from build123d import *

# Parameters (mm, degrees)
F0_R     = 3.175
F0_R_2   = 20.32
F1_DEPTH = 6.35
F2_R     = 7.62
F3_R     = 26.9875
F3_R_2   = 19.685
F4_DEPTH = 12.7
F5_R     = 0.508


with BuildPart() as f1:
    # F0 (on Top) → F1 (new body)
    with BuildSketch(Plane.XY):
        with BuildLine():
            ThreePointArc((-11.5499308761, 24.3910691239), (-8.0975226707, 25.7440339273), (-4.4922459427, 26.6109917636))
            ThreePointArc((-4.4922459427, 26.6109917636), (-5.8575862517, 27.8922864976), (-6.8692513658, 29.4678511747))
            Line((-6.8692513658, 29.4678511747), (-11.5499308761, 24.3910691239))
        make_face()
        with BuildLine():
            ThreePointArc((4.4922459427, 26.6109917636), (8.0975226707, 25.7440339273), (11.5499308761, 24.3910691239))
            Line((11.5499308761, 24.3910691239), (6.8692513658, 29.4678511747))
            ThreePointArc((6.8692513658, 29.4678511747), (5.8575862517, 27.8922864976), (4.4922459427, 26.6109917636))
        make_face()
        with BuildLine():
            ThreePointArc((-4.4922459427, 26.6109917636), (0, 26.9875), (4.4922459427, 26.6109917636))
            ThreePointArc((4.4922459427, 26.6109917636), (5.8575862517, 27.8922864976), (6.8692513658, 29.4678511747))
            ThreePointArc((6.8692513658, 29.4678511747), (7.4299426447, 31.0747423921), (7.62, 32.766))
            ThreePointArc((7.62, 32.766), (-1.6912576079, 40.1959426447), (-6.8692513658, 29.4678511747))
            ThreePointArc((-6.8692513658, 29.4678511747), (-5.8575862517, 27.8922864976), (-4.4922459427, 26.6109917636))
        make_face()
        with Locations((0, 32.766)):
            Circle(F0_R, mode=Mode.SUBTRACT)
        with BuildLine():
            ThreePointArc((-4.4922459427, 26.6109917636), (0, 25.146), (4.4922459427, 26.6109917636))
            ThreePointArc((4.4922459427, 26.6109917636), (0, 26.9875), (-4.4922459427, 26.6109917636))
        make_face()
        with BuildLine():
            ThreePointArc((-26.6109917636, 4.4922459427), (-25.7440339273, 8.0975226707), (-24.3910691239, 11.5499308761))
            Line((-24.3910691239, 11.5499308761), (-29.4678511747, 6.8692513658))
            ThreePointArc((-29.4678511747, 6.8692513658), (-27.8922864976, 5.8575862517), (-26.6109917636, 4.4922459427))
        make_face()
        with BuildLine():
            ThreePointArc((-26.6109917636, -4.4922459427), (-26.9875, 0), (-26.6109917636, 4.4922459427))
            ThreePointArc((-26.6109917636, 4.4922459427), (-27.8922864976, 5.8575862517), (-29.4678511747, 6.8692513658))
            ThreePointArc((-29.4678511747, 6.8692513658), (-40.386, 0), (-29.4678511747, -6.8692513658))
            ThreePointArc((-29.4678511747, -6.8692513658), (-27.8922864976, -5.8575862517), (-26.6109917636, -4.4922459427))
        make_face()
        with Locations((-32.766, 0)):
            Circle(F0_R, mode=Mode.SUBTRACT)
        with BuildLine():
            ThreePointArc((-25.146, 0), (-25.521499922, 2.3625449454), (-26.6109917636, 4.4922459427))
            ThreePointArc((-26.6109917636, 4.4922459427), (-26.9875, 0), (-26.6109917636, -4.4922459427))
            ThreePointArc((-26.6109917636, -4.4922459427), (-25.521499922, -2.3625449454), (-25.146, 0))
        make_face()
        with BuildLine():
            ThreePointArc((-24.3910691239, -11.5499308761), (-25.7440339273, -8.0975226707), (-26.6109917636, -4.4922459427))
            ThreePointArc((-26.6109917636, -4.4922459427), (-27.8922864976, -5.8575862517), (-29.4678511747, -6.8692513658))
            Line((-29.4678511747, -6.8692513658), (-24.3910691239, -11.5499308761))
        make_face()
        with BuildLine():
            ThreePointArc((-6.8692513658, -29.4678511747), (-5.8575862517, -27.8922864976), (-4.4922459427, -26.6109917636))
            ThreePointArc((-4.4922459427, -26.6109917636), (-8.0975226707, -25.7440339273), (-11.5499308761, -24.3910691239))
            Line((-11.5499308761, -24.3910691239), (-6.8692513658, -29.4678511747))
        make_face()
        with BuildLine():
            ThreePointArc((-4.4922459427, -26.6109917636), (0, -26.9875), (4.4922459427, -26.6109917636))
            ThreePointArc((4.4922459427, -26.6109917636), (0, -25.146), (-4.4922459427, -26.6109917636))
        make_face()
        with BuildLine():
            ThreePointArc((6.3892768918, -28.6137065614), (5.5321425722, -27.5257902179), (4.4922459427, -26.6109917636))
            ThreePointArc((4.4922459427, -26.6109917636), (0, -26.9875), (-4.4922459427, -26.6109917636))
            ThreePointArc((-4.4922459427, -26.6109917636), (-5.8575862517, -27.8922864976), (-6.8692513658, -29.4678511747))
            ThreePointArc((-6.8692513658, -29.4678511747), (-1.6912576079, -40.1959426447), (7.62, -32.766))
            ThreePointArc((7.62, -32.766), (7.3058432065, -30.6005773987), (6.3892768918, -28.6137065614))
        make_face()
        with Locations((0, -32.766)):
            Circle(F0_R, mode=Mode.SUBTRACT)
        with BuildLine():
            ThreePointArc((6.3892768918, -28.6137065614), (5.5321425722, -27.5257902179), (4.4922459427, -26.6109917636))
            ThreePointArc((4.4922459427, -26.6109917636), (0, -26.9875), (-4.4922459427, -26.6109917636))
            ThreePointArc((-4.4922459427, -26.6109917636), (-5.8575862517, -27.8922864976), (-6.8692513658, -29.4678511747))
            ThreePointArc((-6.8692513658, -29.4678511747), (-1.6912576079, -40.1959426447), (7.62, -32.766))
            ThreePointArc((7.62, -32.766), (7.3058432065, -30.6005773987), (6.3892768918, -28.6137065614))
        make_face()
        with Locations((0, -32.766)):
            Circle(F0_R, mode=Mode.SUBTRACT)
        with BuildLine():
            Line((6.3892768918, -28.6137065614), (11.5499308761, -24.3910691239))
            ThreePointArc((11.5499308761, -24.3910691239), (8.0975226707, -25.7440339273), (4.4922459427, -26.6109917636))
            ThreePointArc((4.4922459427, -26.6109917636), (5.5321425722, -27.5257902179), (6.3892768918, -28.6137065614))
        make_face()
        with BuildLine():
            ThreePointArc((29.4678511747, -6.8692513658), (27.8922864976, -5.8575862517), (26.6109917636, -4.4922459427))
            ThreePointArc((26.6109917636, -4.4922459427), (25.7440339273, -8.0975226707), (24.3910691239, -11.5499308761))
            Line((24.3910691239, -11.5499308761), (29.4678511747, -6.8692513658))
        make_face()
        with BuildLine():
            ThreePointArc((29.4678511747, 6.8692513658), (27.8922864976, 5.8575862517), (26.6109917636, 4.4922459427))
            ThreePointArc((26.6109917636, 4.4922459427), (26.8932082176, 2.2539982288), (26.9875, 0))
            ThreePointArc((26.9875, 0), (26.8932082176, -2.2539982288), (26.6109917636, -4.4922459427))
            ThreePointArc((26.6109917636, -4.4922459427), (27.8922864976, -5.8575862517), (29.4678511747, -6.8692513658))
            ThreePointArc((29.4678511747, -6.8692513658), (36.8238631046, -6.4496625512), (40.386, 0))
            ThreePointArc((40.386, 0), (36.8238631046, 6.4496625512), (29.4678511747, 6.8692513658))
        make_face()
        with Locations((32.766, 0)):
            Circle(F0_R, mode=Mode.SUBTRACT)
        with BuildLine():
            ThreePointArc((26.9875, 0), (26.8932082176, 2.2539982288), (26.6109917636, 4.4922459427))
            ThreePointArc((26.6109917636, 4.4922459427), (25.146, 0), (26.6109917636, -4.4922459427))
            ThreePointArc((26.6109917636, -4.4922459427), (26.8932082176, -2.2539982288), (26.9875, 0))
        make_face()
        with BuildLine():
            Line((29.4678511747, 6.8692513658), (24.3910691239, 11.5499308761))
            ThreePointArc((24.3910691239, 11.5499308761), (25.7440339273, 8.0975226707), (26.6109917636, 4.4922459427))
            ThreePointArc((26.6109917636, 4.4922459427), (27.8922864976, 5.8575862517), (29.4678511747, 6.8692513658))
        make_face()
        with BuildLine():
            ThreePointArc((26.6109917636, 4.4922459427), (25.7440339273, 8.0975226707), (24.3910691239, 11.5499308761))
            ThreePointArc((24.3910691239, 11.5499308761), (19.0830442573, 19.0830442573), (11.5499308761, 24.3910691239))
            ThreePointArc((11.5499308761, 24.3910691239), (8.0975226707, 25.7440339273), (4.4922459427, 26.6109917636))
            ThreePointArc((4.4922459427, 26.6109917636), (0, 25.146), (-4.4922459427, 26.6109917636))
            ThreePointArc((-4.4922459427, 26.6109917636), (-8.0975226707, 25.7440339273), (-11.5499308761, 24.3910691239))
            ThreePointArc((-11.5499308761, 24.3910691239), (-19.0830442573, 19.0830442573), (-24.3910691239, 11.5499308761))
            ThreePointArc((-24.3910691239, 11.5499308761), (-25.7440339273, 8.0975226707), (-26.6109917636, 4.4922459427))
            ThreePointArc((-26.6109917636, 4.4922459427), (-25.521499922, 2.3625449454), (-25.146, 0))
            ThreePointArc((-25.146, 0), (-25.521499922, -2.3625449454), (-26.6109917636, -4.4922459427))
            ThreePointArc((-26.6109917636, -4.4922459427), (-25.7440339273, -8.0975226707), (-24.3910691239, -11.5499308761))
            ThreePointArc((-24.3910691239, -11.5499308761), (-19.0830442573, -19.0830442573), (-11.5499308761, -24.3910691239))
            ThreePointArc((-11.5499308761, -24.3910691239), (-8.0975226707, -25.7440339273), (-4.4922459427, -26.6109917636))
            ThreePointArc((-4.4922459427, -26.6109917636), (0, -25.146), (4.4922459427, -26.6109917636))
            ThreePointArc((4.4922459427, -26.6109917636), (8.0975226707, -25.7440339273), (11.5499308761, -24.3910691239))
            ThreePointArc((11.5499308761, -24.3910691239), (19.0830442573, -19.0830442573), (24.3910691239, -11.5499308761))
            ThreePointArc((24.3910691239, -11.5499308761), (25.7440339273, -8.0975226707), (26.6109917636, -4.4922459427))
            ThreePointArc((26.6109917636, -4.4922459427), (25.146, 0), (26.6109917636, 4.4922459427))
        make_face()
        Circle(F0_R_2, mode=Mode.SUBTRACT)
        with BuildLine():
            ThreePointArc((-4.4922459427, 26.6109917636), (0, 26.9875), (4.4922459427, 26.6109917636))
            ThreePointArc((4.4922459427, 26.6109917636), (5.8575862517, 27.8922864976), (6.8692513658, 29.4678511747))
            ThreePointArc((6.8692513658, 29.4678511747), (7.4299426447, 31.0747423921), (7.62, 32.766))
            ThreePointArc((7.62, 32.766), (-1.6912576079, 40.1959426447), (-6.8692513658, 29.4678511747))
            ThreePointArc((-6.8692513658, 29.4678511747), (-5.8575862517, 27.8922864976), (-4.4922459427, 26.6109917636))
        make_face()
        with Locations((0, 32.766)):
            Circle(F0_R, mode=Mode.SUBTRACT)
        with BuildLine():
            ThreePointArc((-26.6109917636, -4.4922459427), (-26.9875, 0), (-26.6109917636, 4.4922459427))
            ThreePointArc((-26.6109917636, 4.4922459427), (-27.8922864976, 5.8575862517), (-29.4678511747, 6.8692513658))
            ThreePointArc((-29.4678511747, 6.8692513658), (-40.386, 0), (-29.4678511747, -6.8692513658))
            ThreePointArc((-29.4678511747, -6.8692513658), (-27.8922864976, -5.8575862517), (-26.6109917636, -4.4922459427))
        make_face()
        with Locations((-32.766, 0)):
            Circle(F0_R, mode=Mode.SUBTRACT)
        with BuildLine():
            ThreePointArc((29.4678511747, 6.8692513658), (27.8922864976, 5.8575862517), (26.6109917636, 4.4922459427))
            ThreePointArc((26.6109917636, 4.4922459427), (26.8932082176, 2.2539982288), (26.9875, 0))
            ThreePointArc((26.9875, 0), (26.8932082176, -2.2539982288), (26.6109917636, -4.4922459427))
            ThreePointArc((26.6109917636, -4.4922459427), (27.8922864976, -5.8575862517), (29.4678511747, -6.8692513658))
            ThreePointArc((29.4678511747, -6.8692513658), (36.8238631046, -6.4496625512), (40.386, 0))
            ThreePointArc((40.386, 0), (36.8238631046, 6.4496625512), (29.4678511747, 6.8692513658))
        make_face()
        with Locations((32.766, 0)):
            Circle(F0_R, mode=Mode.SUBTRACT)
        with BuildLine():
            ThreePointArc((6.3892768918, -28.6137065614), (5.5321425722, -27.5257902179), (4.4922459427, -26.6109917636))
            ThreePointArc((4.4922459427, -26.6109917636), (0, -26.9875), (-4.4922459427, -26.6109917636))
            ThreePointArc((-4.4922459427, -26.6109917636), (-5.8575862517, -27.8922864976), (-6.8692513658, -29.4678511747))
            ThreePointArc((-6.8692513658, -29.4678511747), (-1.6912576079, -40.1959426447), (7.62, -32.766))
            ThreePointArc((7.62, -32.766), (7.3058432065, -30.6005773987), (6.3892768918, -28.6137065614))
        make_face()
        with Locations((0, -32.766)):
            Circle(F0_R, mode=Mode.SUBTRACT)
    extrude(amount=F1_DEPTH)

    # F2
    f2_edges = [f1.edges().sort_by_distance(p)[0] for p in [
        (-6.869251, 29.467851, 3.175),
        (-29.467851, 6.869251, 3.175),
        (-29.467851, -6.869251, 3.175),
        (-24.391069, -11.549931, 3.175),
        (-11.549931, -24.391069, 3.175),
        (-6.869251, -29.467851, 3.175),
        (6.389277, -28.613707, 3.175),
        (11.549931, -24.391069, 3.175),
        (24.391069, -11.549931, 3.175),
        (29.467851, -6.869251, 3.175),
        (29.467851, 6.869251, 3.175),
        (24.391069, 11.549931, 3.175),
        (11.549931, 24.391069, 3.175),
        (6.869251, 29.467851, 3.175),
        (-11.549931, 24.391069, 3.175),
        (-24.391069, 11.549931, 3.175),
    ]]
    fillet(f2_edges, radius=F2_R)

    # F3 (on Top) → F4 (join)
    with BuildSketch(Plane.XY):
        Circle(F3_R)
        Circle(F3_R_2, mode=Mode.SUBTRACT)
    extrude(amount=F4_DEPTH)

    # F5
    f5_edges = [f1.edges().sort_by_distance(p)[0] for p in [
        (-19.685, 0, 12.7),
        (-19.685, 0, 0),
    ]]
    fillet(f5_edges, radius=F5_R)


solid = f1.part
Part model, mm, in its own coordinate system. Give positions to 0.01 mm unless a question says otherwise; leave off trailing zeros. Write each loop counter-clockwise with the first axis right and the second up, starting at its lowest first coordinate (ties: lowest second). Pieces come first, ordered by that corner, then holes.
1) Pin check, flat tips, straight feed: pin 1 (7.5 mm diameter, centred on x = 0, y = -32.766, fed in from +Z); pin 2 (5 mm diameter, centred on y = 14, z = 6, fed in from +X); pin 3 (6 mm diameter, centred on x = 31.5, z = 5.5, fed in from +Y). Stop position of each tip, or through.
Resolved:
pin 1: stops at z = 6.35
pin 2: stops at x = 24.59
pin 3: stops at y = 8.27
2) Cut at B-B on x = 35. Write the cut outline in (y, z).
Resolved:
outline: (-7.29, 0) - (-2.26, 0) - (-2.26, 6.35) - (-7.29, 6.35) - close; (2.26, 0) - (7.29, 0) - (7.29, 6.35) - (2.26, 6.35) - close
3) Cut at A-A on x = 0. State how many separate pieces and enclosed holes the cut face has, then the cut area to 3 significant figures.
Resolved:
separate pieces: 4
enclosed holes: 0
area: 275 mm2
4) Two-plate mould, pull along X, no slides. Class faces 1 (the face through (-35.938, 0.14, 3.131)), 2 (the face through (-11.55, -24.55, 3.22)), 3 (the face through (30, -3, 6.35)): released by +X, released by -X, zero draft, split by the parting line, or undercut.
Resolved:
face 1: undercut
face 2: released by -X
face 3: zero draft
5) Probe L1, parallel to Y at x = 0, z = 2 (3 decimals); L2, parallel to Y at x = 10, z = 8.5; L3, parallel to X at y = -34.5, z = 4.75. List the from-to ranges inside material, lowest first.
Resolved:
L1: y = -40.386 to -35.941, -29.591 to -19.685, 19.685 to 29.591, 35.941 to 40.386
L2: y = -25.07 to -16.96, 16.96 to 25.07
L3: x = -7.42 to -2.66, 2.66 to 7.42
6) Cut at C-C on z = 9. Write the cut outline in (x, y) (1 decimal), then the cut area to 3 significant figures.
Resolved:
outline: circle Ø54 at (0, 0); hole circle Ø39.4 at (0, 0)
area: 1,070 mm2
